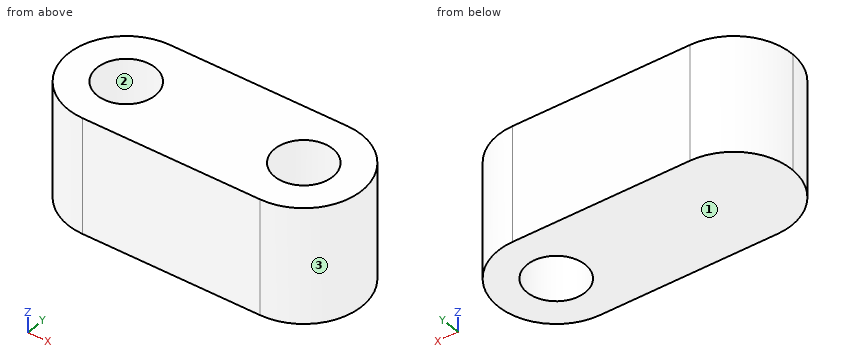
from build123d import *

# Parameters (mm, degrees)
F0_R     = 3
F1_DEPTH = 12
F2_R     = 3
F3_DEPTH = 6.9


with BuildPart() as f1:
    # F0 (on Top) → F1 (new body)
    with BuildSketch(Plane.XY):
        with BuildLine():
            Line((-40, 12), (-58, 12))
            ThreePointArc((-58, 12), (-62.242641, 10.242641), (-64, 6))
            ThreePointArc((-64, 6), (-62.242641, 1.757359), (-58, 0))
            Line((-58, 0), (-40, 0))
            ThreePointArc((-40, 0), (-34, 6), (-40, 12))
        make_face()
        with Locations((-40, 6)):
            Circle(F0_R, mode=Mode.SUBTRACT)
    extrude(amount=F1_DEPTH)

    # F2 (on face) → F3 (cut)
    with BuildSketch(Plane.XY.offset(12)):
        with Locations((-58, 6)):
            Circle(F2_R)
    extrude(amount=-F3_DEPTH, mode=Mode.SUBTRACT)


solid = f1.part
The model under review builds one solid part; all positions refer to its coordinate system, in mm. Face numbers are marked on the shaded views. Coordinates: 2 decimals unless noted, no trailing zeros. Order: outer loops, then holes, each group sorted by start corner. A loop starts at its lowest first (then second) coordinate and runs counter-clockwise, first axis right, second up. Notation, with made-up numbers: (85, 64) -> (133, 64) arc R20 ccw to (133, 83) -> close; hole circle Ø4 at (48, 30.5). An arc over 180 degrees is marked (long way). Answer in a Markdown table with one row per item.
(1) Insertion check: pin 1 (6 mm diameter, centred on y = 2.5, z = 10, fed in from -X); pin 2 (1.5 mm diameter, centred on y = 9.5, z = 7, fed in from -X); pin 3 (1.8 mm diameter, centred on x = -57.5, y = 6.5, fed in from +Z); pin 4 (3.5 mm diameter, centred on x = -40, y = 6, fed in from +Z). Each pin has a flat end and moves straight along its axis. Give the tip position at first contact, or say it passes through.
Answers:
| item | result |
|---|---|
| pin 1 | x = -63.98 |
| pin 2 | x = -63.33 |
| pin 3 | z = 5.1 |
| pin 4 | through |
(2) Wall thickness on line 1 along Y through (x, z) = (-58, 10); line 2 along X through (y, z) = (5, 5.5); line 3 along X through (y, z) = (3.75, 5.5): over which ranges is each line inside the solid? List them lowest first.
Answers:
| item | result |
|---|---|
| line 1 | 0 to 3, 9 to 12 |
| line 2 | -63.92 to -60.83, -55.17 to -42.83, -37.17 to -34.08 |
| line 3 | -63.56 to -59.98, -56.02 to -41.98, -38.02 to -34.44 |
(3) The part is to be moulded in two halves that separate along X. For the marked faces 1, 2 and 3, say which applies: +X half, -X half, draft (parallel to the pull), parting line (faces both ways), or undercut.
Answers:
| item | result |
|---|---|
| face 1 | draft |
| face 2 | undercut |
| face 3 | +X half |
(4) Consider section D-D (x = -56). Write out the cut boundary in (y, z).
Answers:
| item | result |
|---|---|
| outline | (0, 0) -> (12, 0) -> (12, 12) -> (8.24, 12) -> (8.24, 5.1) -> (3.76, 5.1) -> (3.76, 12) -> (0, 12) -> close |
(5) Consider section A-A (z = 5.5). Write out the cut boundary in (x, y), plus the area to 3 significant figures.
Answers:
| item | result |
|---|---|
| outline | (-64, 6) arc R6 ccw to (-58, 0) -> (-40, 0) arc R6 ccw to (-40, 12) -> (-58, 12) arc R6 ccw to start; hole circle Ø6 at (-58, 6); hole circle Ø6 at (-40, 6) |
| area | 273 mm² |
(6) Consider section B-B (y = 8.25). Write out the cut boundary in (x, z).
Answers:
| item | result |
|---|---|
| outline | (-63.56, 0) -> (-41.98, 0) -> (-41.98, 12) -> (-56.02, 12) -> (-56.02, 5.1) -> (-59.98, 5.1) -> (-59.98, 12) -> (-63.56, 12) -> close; (-38.02, 0) -> (-34.44, 0) -> (-34.44, 12) -> (-38.02, 12) -> close |
(7) Consider section C-C (z = 2). Write out the cut boundary in (x, y), plus the area to 3 significant figures.
Answers:
| item | result |
|---|---|
| outline | (-64, 6) arc R6 ccw to (-58, 0) -> (-40, 0) arc R6 ccw to (-40, 12) -> (-58, 12) arc R6 ccw to start; hole circle Ø6 at (-40, 6) |
| area | 301 mm² |
